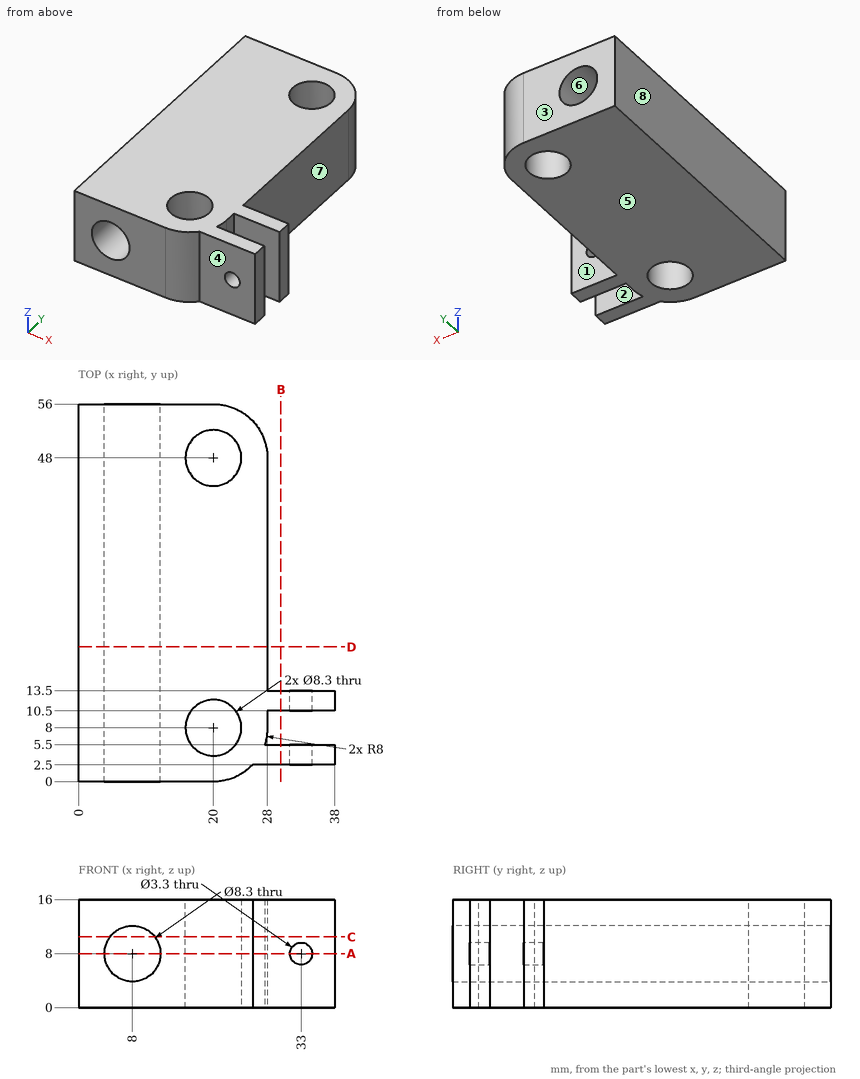
Design review of the part shown in the three views and the two pictorial views. Dimensions are in mm from the part's minimum x, y and z. A direction names the side the tool comes from. Round coordinates to 2 decimals unless told otherwise and drop trailing zeros. Loops run counter-clockwise (first coordinate to the right, second up) from the corner with the lowest first, then second, coordinate; pieces in that order, holes last. Notation, with made-up numbers: (80.25, 9.5) -> (130.25, 9.5) arc R29 cw to (130.25, 43.5) -> close; hole circle Ø2 at (22.5, 24). An arc over 180 degrees is marked (long way). Use one line per item in the form item = value. Start each with the question number.
Q1. We need section B-B on x = 30. Give the boundary of the cut face in (y, z).
Q2. Machinability: for the marked faces 1, 2, 3 and 4, which of the approach directions +Z, -Z, +X, -X, +Y, -Y give a long, thin tool a straight path to every point of the face, cutting with its end or side? Answer none if there is none.
Q3. Draft analysis for pull direction X (two halves, no side actions). For the marked faces 5, 6, 7 and 8, state which applies: +X half, -X half, draft (parallel to the pull), parting line (faces both ways), or undercut.
Q4. We need section D-D on y = 20. Give the boundary of the cut face in (x, z).
Q5. For pin 1 Ø3 at (x, z) = (31.5, 5) entering from -Y; pin 2 Ø11 at (x, y) = (20, 48) entering from -Z; pin 3 Ø2 at (y, z) = (9, 9.5) entering from +X; pin 4 Ø6.5 at (x, y) = (20, 8) entering from -Z, all flat-tipped, find the tip position at first contact; note any pin that passes through.
Q6. Wall thickness on line 1 along Y through (x, z) = (20, 8); line 2 along X through (y, z) = (12.95, 8); line 3 along Y through (x, z) = (36, 4): over which ranges is each line inside the solid? List them lowest first. Write a range as [from, to].
Q7. We need section C-C on z = 10.5. Give the boundary of the cut face in (x, y), then the cut area to 3 significant figures.
Q8. We need section A-A on z = 8. Give the boundary of the cut face in (x, y), then the cut area to 3 significant figures.
Calculated:
q1.outline = (2.5, 0) -> (5.5, 0) -> (5.5, 16) -> (2.5, 16) -> close; (10.5, 0) -> (13.5, 0) -> (13.5, 16) -> (10.5, 16) -> close
q2.face_1 = +Z, -Z, +X, +Y
q2.face_2 = +Z, -Z, +X
q2.face_3 = +Z, -Z, +X, -X, +Y
q2.face_4 = +Z, -Z, +X, -Y
q3.face_5 = draft
q3.face_6 = undercut
q3.face_7 = +X half
q3.face_8 = -X half
q4.outline = (0, 0) -> (28, 0) -> (28, 16) -> (0, 16) -> close; hole circle Ø8.3 at (8, 8)
q5.pin_1 = 2.5
q5.pin_2 = 0
q5.pin_3 = 28
q5.pin_4 = through
q6.line_1 = [0, 3.85], [12.15, 43.85], [52.15, 56]
q6.line_2 = [0, 3.85], [12.15, 31.35], [34.65, 38]
q6.line_3 = [2.5, 5.5], [10.5, 13.5]
q7.outline = (0, 0) -> (4.69, 0) -> (4.69, 56) -> (0, 56) -> close; (11.31, 0) -> (20, 0) arc R8 ccw to (25.81, 2.5) -> (38, 2.5) -> (38, 5.5) -> (27.6, 5.5) arc R8 ccw to (28, 8) -> (28, 10.5) -> (38, 10.5) -> (38, 13.5) -> (28, 13.5) -> (28, 48) arc R8 ccw to (20, 56) -> (11.31, 56) -> close; hole circle Ø8.3 at (20, 8); hole circle Ø8.3 at (20, 48)
q7.area = 1,120 mm²
q8.outline = (0, 0) -> (3.85, 0) -> (3.85, 56) -> (0, 56) -> close; (12.15, 0) -> (20, 0) arc R8 ccw to (25.81, 2.5) -> (31.35, 2.5) -> (31.35, 5.5) -> (27.6, 5.5) arc R8 ccw to (28, 8) -> (28, 10.5) -> (31.35, 10.5) -> (31.35, 13.5) -> (28, 13.5) -> (28, 48) arc R8 ccw to (20, 56) -> (12.15, 56) -> close; (34.65, 2.5) -> (38, 2.5) -> (38, 5.5) -> (34.65, 5.5) -> close; (34.65, 10.5) -> (38, 10.5) -> (38, 13.5) -> (34.65, 13.5) -> close; hole circle Ø8.3 at (20, 8); hole circle Ø8.3 at (20, 48)
q8.area = 1,010 mm²
